from build123d import *

# Parameters (mm, degrees)
SKETCH1_R           = 57.5
BOSS_EXTRUDE1_DEPTH = 33.6
SKETCH2_R           = 50
CUT_EXTRUDE1_DEPTH  = 28.6
FILLET1_R           = 5
SKETCH3_W           = 40
SKETCH3_H           = 22.6
CUT_EXTRUDE2_DEPTH  = 88.985566998
CIRPATTERN1_COUNT   = 3


with BuildPart() as part:
    # Sketch1 → Boss-Extrude1 (new body)
    with BuildSketch(Plane(origin=(0, 0, 0), x_dir=(1, 0, 0), z_dir=(0, 1, 0))):
        with Locations(Location((0, 0, 0), (0, 0, 270))):
            Circle(SKETCH1_R)
    extrude(amount=BOSS_EXTRUDE1_DEPTH)

    # Sketch2 → Cut-Extrude1 (cut)
    with BuildSketch(Plane(origin=(0, 33.6, 0), x_dir=(1, 0, 0), z_dir=(0, 1, 0))):
        with Locations(Location((0, 0, 0), (0, 0, 270))):
            Circle(SKETCH2_R)
    extrude(amount=-CUT_EXTRUDE1_DEPTH, mode=Mode.SUBTRACT)

    # Fillet1
    fillet1_edges = [part.edges().sort_by_distance(p)[0] for p in [
        (0, 5, -50),
    ]]
    fillet(fillet1_edges, radius=FILLET1_R)

    # Sketch3 → Cut-Extrude2 (cut, symmetric)
    with BuildSketch(Plane.XY):
        with Locations((0, 16.3)):
            Rectangle(SKETCH3_W, SKETCH3_H)
    cut_extrude2 = extrude(amount=CUT_EXTRUDE2_DEPTH, both=True, mode=Mode.SUBTRACT)

    # CirPattern1: Cut-Extrude2 ×3 about axis
    cirpattern1_axis = Axis((0, 0, 0), (0, 1, 0))
    for i in range(1, CIRPATTERN1_COUNT):
        add(cut_extrude2.rotate(cirpattern1_axis, i * 360 / CIRPATTERN1_COUNT), mode=Mode.SUBTRACT)


solid = part.part
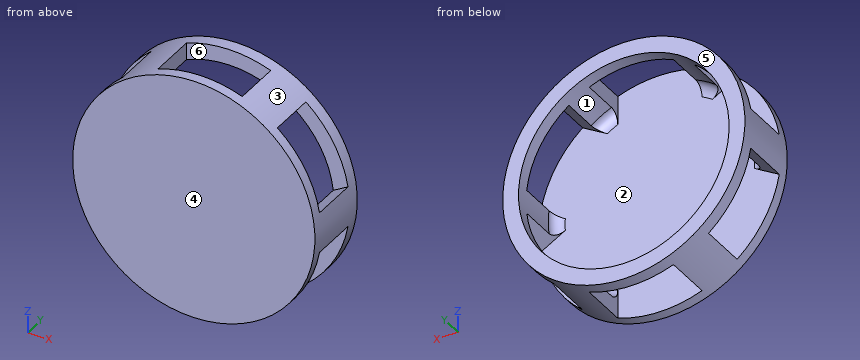
Could you check a few things on this model? Use its own coordinates, in mm. Face numbers are marked on the shaded views. A direction names the side the tool comes from. Round coordinates to 2 decimals unless told otherwise and drop trailing zeros. Write each loop counter-clockwise with the first axis right and the second up, starting at its lowest first coordinate (ties: lowest second). Pieces come first, ordered by that corner, then holes. Notation, with made-up numbers: (-21.75, 23) -> (-14.75, 23) arc R20 ccw to (-14.75, 30) -> close; hole circle Ø11 at (25, 74). An arc over 180 degrees is marked (long way). Use a Markdown table: item, result.
1. We'd pull the mould along Y, two halves only. Please class the marked faces 4, 5 and 6: +Y half, -Y half, draft (parallel to the pull), parting line (faces both ways), or undercut.
Answer key:
| item | result |
|---|---|
| face 4 | -Y half |
| face 5 | +Y half |
| face 6 | undercut |
2. Which directions (+Z, -Z, +X, -X, +Y, -Y) give clear straight access to the entire face, cutting with the end or side of a thin tool? Please do the marked faces 1, 2 and 3.
Answer key:
| item | result |
|---|---|
| face 1 | +Y |
| face 2 | none |
| face 3 | +Y, -Y |
3. For pin 1 Ø6 at (x, y) = (-36.5, 21) entering from +Z; pin 2 Ø3 at (y, z) = (20, -41) entering from +X; pin 3 Ø11 at (y, z) = (20, -47.5) entering from +X; pin 4 Ø4 at (x, y) = (11, 25.5) entering from -Z, each with a flat end and sliding along its axis, tell me the tip position at first contact or that it passes through.
Answer key:
| item | result |
|---|---|
| pin 1 | stops at z = 46.73 |
| pin 2 | stops at x = 33.61 |
| pin 3 | stops at x = 36.69 |
| pin 4 | passes through |
4. If we section it at A-A (x = 0): List the corners of the cut face in (y, z) for me, then the cut area to 3 significant figures.
Answer key:
| item | result |
|---|---|
| outline | (0, -57.5) -> (5, -57.5) -> (5, 57.5) -> (0, 57.5) -> close; (27.6, -57.5) -> (33.6, -57.5) -> (33.6, -50) -> (27.6, -50) -> close; (27.6, 50) -> (33.6, 50) -> (33.6, 57.5) -> (27.6, 57.5) -> close |
| area | 665 mm^2 |
5. If we section it at D-D (y = 17): List the corners of the cut face in (x, z) for me.
Answer key:
| item | result |
|---|---|
| outline | (-56.69, -9.63) -> (-49.69, -5.59) arc R50 cw to (-49.69, 5.59) -> (-56.69, 9.63) arc R57.5 ccw to start; (-36.69, -44.28) arc R57.5 ccw to (-20, -53.91) -> (-20, -45.83) arc R50 cw to (-29.69, -40.23) -> close; (-36.69, 44.28) -> (-29.69, 40.23) arc R50 cw to (-20, 45.83) -> (-20, 53.91) arc R57.5 ccw to start; (20, -53.91) arc R57.5 ccw to (36.69, -44.28) -> (29.69, -40.23) arc R50 cw to (20, -45.83) -> close; (20, 45.83) arc R50 cw to (29.69, 40.23) -> (36.69, 44.28) arc R57.5 ccw to (20, 53.91) -> close; (49.69, -5.59) -> (56.69, -9.63) arc R57.5 ccw to (56.69, 9.63) -> (49.69, 5.59) arc R50 cw to start |
6. If we section it at C-C (y = 29): List the corners of the cut face in (x, z) for me, then the cut area to 3 significant figures.
Answer key:
| item | result |
|---|---|
| outline | circle Ø115 at (0, 0); hole circle Ø100 at (0, 0) |
| area | 2,530 mm^2 |
7. Please list where these lines run through material, in increasing order: probe 1 along X at (y, z) = (24, 0); probe 2 along Z at (x, y) = (1.5, 31.5); probe 3 along Y at (x, z) = (-47, 29).
Answer key:
| item | result |
|---|---|
| probe 1 | x = -57.5 to -50, 50 to 57.5 |
| probe 2 | z = -57.48 to -49.98, 49.98 to 57.48 |
| probe 3 | y = 0 to 5, 27.6 to 33.6 |
8. If we section it at B-B (z = 0): List the corners of the cut face in (x, y) for me.
Answer key:
| item | result |
|---|---|
| outline | (-57.5, 0) -> (57.5, 0) -> (57.5, 33.6) -> (50, 33.6) -> (50, 10) arc R5 cw to (45, 5) -> (-45, 5) arc R5 cw to (-50, 10) -> (-50, 33.6) -> (-57.5, 33.6) -> close |
